Input: dimensioned drawing with shaded views. Units: mm. Origin: part minimum x, y, z. A direction names the side the tool comes from. Round coordinates to 2 decimals unless told otherwise and drop trailing zeros. Loops run counter-clockwise (first coordinate to the right, second up) from the corner with the lowest first, then second, coordinate; pieces in that order, holes last. Notation, with made-up numbers: M 78,55.25 L 113,55.25 A15 ccw 113,72.25 Z; hole C -25,-37.5 d6. An arc over 180 degrees is marked long. Write each question's results on one line, items separated by ' | '. Start each with the question number.
1. Draft query along Y for the marked faces 3 and 4. Return one class per face: released by +Y, released by -Y, zero draft, split by the parting line, or undercut.
2. Ray query, line 1 (X direction, y = 26.5, z = 6) (1 decimal); line 2 (Z direction, x = 34, y = 7.5); line 3 (Y direction, x = 26, z = 6.5) (1 decimal). Return the intervals inside material, ascending.
3. Section A-A on z = 5.75. Output: boundary loops of the cut face in (x, y), and give its area (3 significant figures).
4. Set-up query: the marked faces 1 and 2. Return all of +Z, -Z, +X, -X, +Y, -Y with unobstructed straight access to the full face (end or side cutting, diameter ignored); none if empty.
5. Section B-B on y = 19.8. Output: boundary loops of the cut face in (x, z).
6. Section C-C on x = 5. Output: boundary loops of the cut face in (y, z), and give its area (3 significant figures).
7. Contact query for flat-ended pins moving along their axis: pin 1 Ø1.5 at (x, z) = (19, 2) entering from +Y; pin 2 Ø4 at (x, z) = (23.5, 1) entering from -Y; pin 3 Ø1 at (x, z) = (17.5, 2.5) entering from +Y. Output: stop coordinate, or through.
8. Section D-D on z = 3.5. Output: boundary loops of the cut face in (x, y).
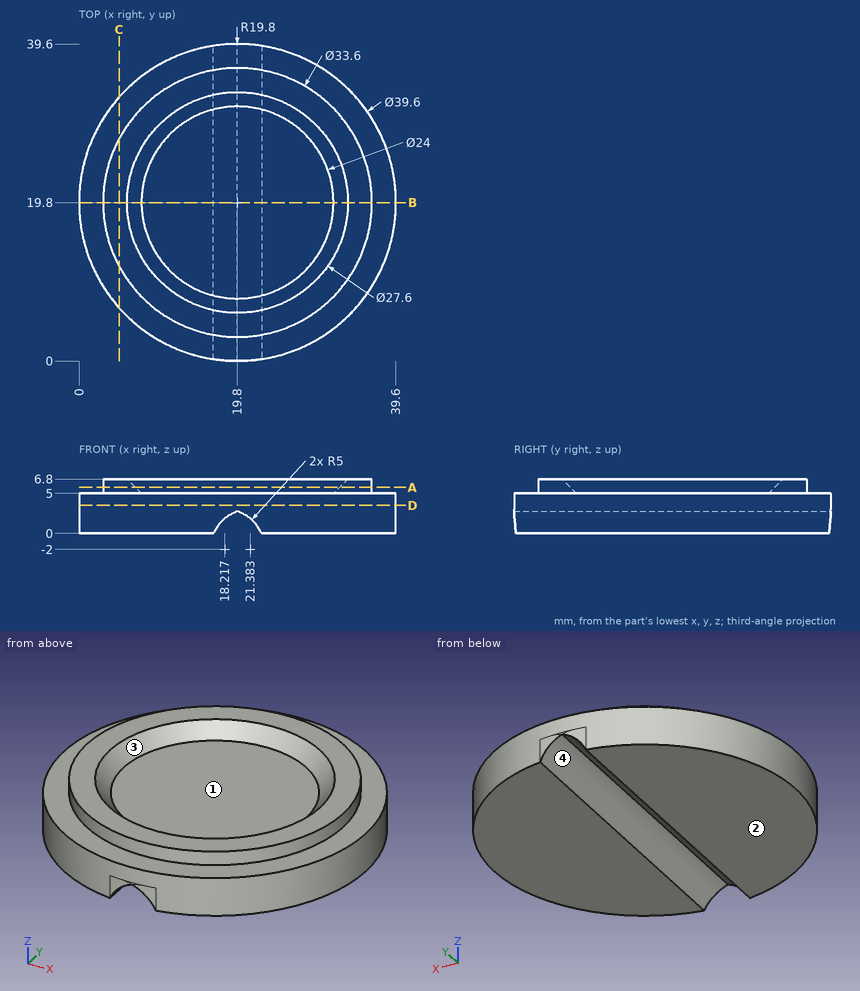
Taken from the geometry:
1) face 3: undercut | face 4: zero draft
2) line 1: 4.4 to 8.7, 30.9 to 35.2 | line 2: 0 to 5 | line 3: 4.2 to 7.8, 31.8 to 35.4
3) outline: C 19.8,19.8 d33.6; hole C 19.8,19.8 d25.5 | area: 376 mm^2
4) face 1: +Z | face 2: -Z, +X, -X, +Y, -Y
5) outline: M 0,0 L 16.8,0 A5 cw 19.8,2.74 A5 cw 22.8,0 L 39.6,0 L 39.6,5 L 36.6,5 L 36.6,6.8 L 33.6,6.8 L 31.8,5 L 7.8,5 L 6,6.8 L 3,6.8 L 3,5 L 0,5 Z
6) outline: M 6.65,0 L 32.95,0 L 32.95,5 L 27.75,5 L 27.75,6.8 L 11.85,6.8 L 11.85,5 L 6.65,5 Z | area: 160 mm^2
7) pin 1: y = 39.6 | pin 2: y = 0.08 | pin 3: y = 39.52
8) outline: C 19.8,19.8 d39.6
